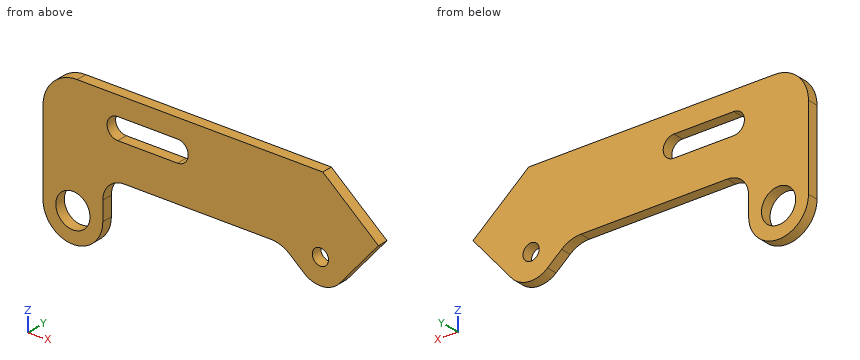
```python
from build123d import *

# Parameters (mm, degrees)
F0_R     = 8
F0_R_2   = 3.8
F1_DEPTH = 5
F2_R     = 10
F3_R     = 14
F4_R     = 16


with BuildPart() as f1:
    # F0 (on Front) → F1 (new body)
    with BuildSketch(Plane.XZ):
        with BuildLine():
            Line((38.056332, 55), (-92.943668, 55))
            Line((-92.943668, 55), (-92.943668, 0))
            ThreePointArc((-92.943668, 0), (-78.943668, -14), (-64.943668, 0))
            Line((-64.943668, 0), (-64.943668, 19))
            Line((-64.943668, 19), (18.730509, 19))
            Line((18.730509, 19), (29.202295, 10.213128))
            ThreePointArc((29.202295, 10.213128), (37.961615, 7.451325), (46.108279, 11.69221))
            Line((46.108279, 11.69221), (64.106332, 33.141455))
            Line((64.106332, 33.141455), (38.056332, 55))
        make_face()
        with Locations((-78.943668, 0)):
            Circle(F0_R, mode=Mode.SUBTRACT)
        with Locations((36.915746, 19.405662)):
            Circle(F0_R_2, mode=Mode.SUBTRACT)
        with BuildLine():
            ThreePointArc((-57.943668, 36), (-62.943668, 41), (-57.943668, 46))
            Line((-57.943668, 46), (-29.943668, 46))
            ThreePointArc((-29.943668, 46), (-24.943668, 41), (-29.943668, 36))
            Line((-29.943668, 36), (-57.943668, 36))
        make_face(mode=Mode.SUBTRACT)
    extrude(amount=F1_DEPTH)

    # F2
    f2_edges = [f1.edges().sort_by_distance(p)[0] for p in [
        (-64.943668, -2.5, 19),
    ]]
    fillet(f2_edges, radius=F2_R)

    # F3
    f3_edges = [f1.edges().sort_by_distance(p)[0] for p in [
        (18.730509, -2.5, 19),
    ]]
    fillet(f3_edges, radius=F3_R)

    # F4
    f4_edges = [f1.edges().sort_by_distance(p)[0] for p in [
        (-92.943668, -2.5, 55),
    ]]
    fillet(f4_edges, radius=F4_R)


solid = f1.part
```
Read the model definition and answer for the solid it produces. Units are mm, in the model's axes. Coordinates: 2 decimals unless noted, no trailing zeros. Loops run counter-clockwise (first coordinate to the right, second up) from the corner with the lowest first, then second, coordinate; pieces in that order, holes last.
(1) Flat-ended cylindrical pins translate along their axes: pin 1 Ø1 at (y, z) = (-0.5, 2) entering from +X; pin 2 Ø6 at (x, z) = (-64.5, -6) entering from -Y; pin 3 Ø1.5 at (x, y) = (-44.5, -1.5) entering from -Z. Find the tip coordinate at first contact, or state that the pin passes through.
Solution:
pin 1: stops at x = -64.94
pin 2: stops at y = -5
pin 3: stops at z = 19
(2) The part is cut by section B-B (y = -3). Determine the outline of the cut face in (x, z), and give its area (3 significant figures).
Solution:
outline: (-92.94, 0) arc R14 ccw to (-64.94, 0) - (-64.94, 9) arc R10 cw to (-54.94, 19) - (13.63, 19) arc R14 cw to (22.63, 15.72) - (29.2, 10.21) arc R12 ccw to (46.11, 11.69) - (64.11, 33.14) - (38.06, 55) - (-76.94, 55) arc R16 ccw to (-92.94, 39) - close; hole circle Ø16 at (-78.94, 0); hole (-57.94, 36) - (-29.94, 36) arc R5 ccw to (-29.94, 46) - (-57.94, 46) arc R5 ccw to start; hole circle Ø7.6 at (36.92, 19.41)
area: 5,740 mm2
(3) The part is cut by section C-C (x = -68). Determine the outline of the cut face in (y, z).
Solution:
outline: (-5, -8.73) - (0, -8.73) - (0, 55) - (-5, 55) - close
(4) Consider line 1 along Z through (x, y) = (-38, -3.65); line 2 along X through (y, z) = (-4.25, 17); line 3 along Z through (x, y) = (6, -3.7). Determine where each line is inside the solid, lowest interval first.
Solution:
line 1: z = 19 to 36, 46 to 55
line 2: x = -92.94 to -60.94, 20.85 to 33.97, 39.86 to 50.56
line 3: z = 19 to 55
(5) The part is cut by section A-A (z = 41). Determine the outline of the cut face in (x, y), and give its area (3 significant figures).
Solution:
outline: (-92.82, -5) - (-62.94, -5) - (-62.94, 0) - (-92.82, 0) - close; (-24.94, -5) - (54.74, -5) - (54.74, 0) - (-24.94, 0) - close
area: 548 mm2
